Answer from the drawing. Dimensions are ordinates in mm from the lowest x, y and z of the part. Coordinates: 2 decimals unless noted, no trailing zeros. Order: outer loops, then holes, each group sorted by start corner. A loop starts at its lowest first (then second) coordinate and runs counter-clockwise, first axis right, second up. Notation, with made-up numbers: (-2, 67) - (29, 67) arc R14 cw to (29, 85) - close; hole circle Ø4 at (37.5, 55). An arc over 180 degrees is marked (long way). Use a Markdown table: item, result. Add a question column.
Item 1: Find the intervals of material crossed by line 1 along X through (y, z) = (5, 1.1); line 2 along Z through (x, y) = (6, 7.75), in increasing order.
Item 2: The part is cut by section A-A, the plane x = 5. Give the vertices of the cut face in (y, z), then the cut area to 3 significant figures.
Item 3: The part is cut by section B-B, the plane z = 76.5. Give the vertices of the cut face in (x, y).
Item 4: A flat-ended cylindrical pin translates along its axis: P1, Ø4, axis at x = 5, z = 69.5, coming from the -Y side. Find the tip coordinate at first contact, or state that the pin passes through.
Item 5: The mould has two halves that part along Z. Classify the marked faces 1 and 2: released by +Z, released by -Z, zero draft, split by the parting line, or undercut.
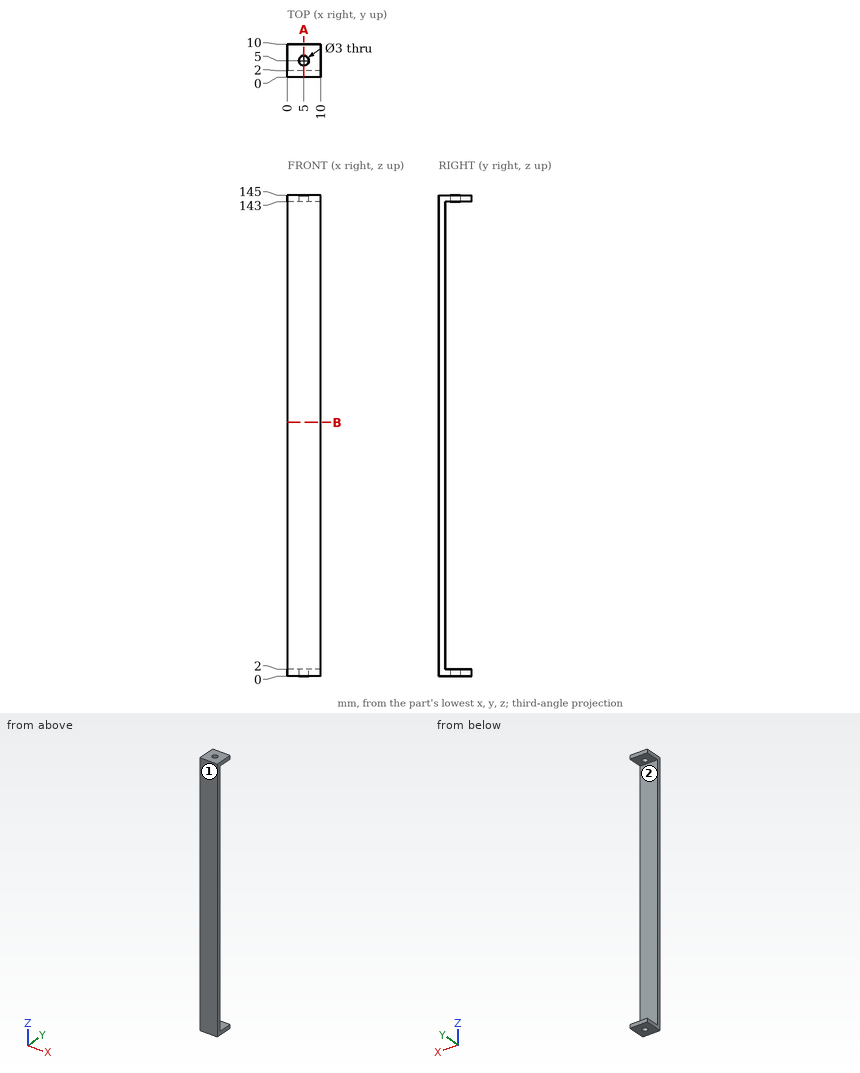
Solution:
| question | item | result |
|---|---|---|
| 1 | line 1 | x = 0 to 3.5, 6.5 to 10 |
| 1 | line 2 | z = 0 to 2, 143 to 145 |
| 2 | outline | (0, 0) - (3.5, 0) - (3.5, 2) - (2, 2) - (2, 143) - (3.5, 143) - (3.5, 145) - (0, 145) - close; (6.5, 0) - (10, 0) - (10, 2) - (6.5, 2) - close; (6.5, 143) - (10, 143) - (10, 145) - (6.5, 145) - close |
| 2 | area | 310 mm2 |
| 3 | outline | (0, 0) - (10, 0) - (10, 2) - (0, 2) - close |
| 4 | P1 | stops at y = 0 |
| 5 | face 1 | zero draft |
| 5 | face 2 | undercut |
